For this review, take the finished solid that the model builds, in its own axes (mm). A direction names the side the tool comes from. Coordinates: 2 decimals unless noted, no trailing zeros. Order: outer loops, then holes, each group sorted by start corner. A loop starts at its lowest first (then second) coordinate and runs counter-clockwise, first axis right, second up.
from build123d import *

# Parameters (mm, degrees)
BOSS_EXTRUDE1_DEPTH = 1.5
SKETCH2_W           = 0.621894726
SKETCH2_H           = 0.5
SKETCH3_W           = 0.313581939
SKETCH3_H           = 0.5
SKETCH4_W           = 0.917270519
SKETCH4_H           = 0.5
SKETCH5_W           = 0.282237083
SKETCH5_H           = 0.5
SKETCH6_W           = 0.605170604
SKETCH6_H           = 0.5


with BuildPart() as part:
    # Sketch1 → Boss-Extrude1 (new body)
    with BuildSketch(Plane(origin=(0, 0, 0), x_dir=(-1, 0, 0), z_dir=(0, 0, -1))):
        with BuildLine():
            Line((3.5, 1.5), (-3.5, 1.5))
            ThreePointArc((-3.5, 1.5), (-5, 0), (-3.5, -1.5))
            Line((-3.5, -1.5), (3.5, -1.5))
            ThreePointArc((3.5, -1.5), (5, 0), (3.5, 1.5))
        make_face()
    extrude(amount=-BOSS_EXTRUDE1_DEPTH)

    # Sketch2 → Revolve1 (revolve)
    with BuildSketch(Plane.XZ, mode=Mode.PRIVATE) as revolve1_sk:
        with Locations((3.731030185, 1.75)):
            Rectangle(SKETCH2_W, SKETCH2_H)
    revolve(revolve1_sk.sketch.rotate(Axis((3.420082822, 0, 2), (0, 0, -1)), 180), axis=Axis((3.420082822, 0, 2), (0, 0, -1)))

    # Sketch3 → Revolve2 (revolve)
    with BuildSketch(Plane.XZ, mode=Mode.PRIVATE) as revolve2_sk:
        with Locations((2.315287044, 1.75)):
            Rectangle(SKETCH3_W, SKETCH3_H)
    revolve(revolve2_sk.sketch.rotate(Axis((2.158496075, 0, 2), (0, 0, -1)), 180), axis=Axis((2.158496075, 0, 2), (0, 0, -1)))

    # Sketch4 → Revolve3 (revolve)
    with BuildSketch(Plane.XZ, mode=Mode.PRIVATE) as revolve3_sk:
        with Locations((0.45863526, 1.75)):
            Rectangle(SKETCH4_W, SKETCH4_H)
    revolve(revolve3_sk.sketch.rotate(Axis((0, 0, 2), (0, 0, -1)), 180), axis=Axis((0, 0, 2), (0, 0, -1)))

    # Sketch5 → Revolve4 (revolve)
    with BuildSketch(Plane.XZ.offset(0.093633391), mode=Mode.PRIVATE) as revolve4_sk:
        with Locations((-1.554138651, 1.75)):
            Rectangle(SKETCH5_W, SKETCH5_H)
    revolve(revolve4_sk.sketch.rotate(Axis((-1.695257192, -0.093633391, 2), (0, 0, -1)), 180), axis=Axis((-1.695257192, -0.093633391, 2), (0, 0, -1)))

    # Sketch6 → Revolve5 (revolve)
    with BuildSketch(Plane.XZ.offset(0.093633391), mode=Mode.PRIVATE) as revolve5_sk:
        with Locations((-2.693683223, 1.75)):
            Rectangle(SKETCH6_W, SKETCH6_H)
    revolve(revolve5_sk.sketch.rotate(Axis((-2.996268525, -0.093633391, 2), (0, 0, -1)), 180), axis=Axis((-2.996268525, -0.093633391, 2), (0, 0, -1)))


solid = part.part
1. Take a section at A-A, the plane x = 0. Give the boundary of the cut face in (y, z).
Answer below:
outline: (-1.5, 0) - (1.5, 0) - (1.5, 1.5) - (0.92, 1.5) - (0.92, 2) - (-0.92, 2) - (-0.92, 1.5) - (-1.5, 1.5) - close
2. Take a section at D-D, the plane x = 1.25. Give the boundary of the cut face in (y, z).
Answer below:
outline: (-1.5, 0) - (1.5, 0) - (1.5, 1.5) - (-1.5, 1.5) - close
3. Take a section at C-C, the plane z = 0.4. Give the boundary of the cut face in (x, y), plus the area to 3 significant figures.
Answer below:
outline: (-3.5, -1.5) - (3.5, -1.5) arc R1.5 ccw to (3.5, 1.5) - (-3.5, 1.5) arc R1.5 ccw to start
area: 28.1 mm2
4. The part is to be moulded in two halves that separate along X. For faces 3 (the face through (-3, 0, 2)), 4 (the face through (-3.573, 0.088, 1.754)), 5 (the face through (5, 0, 1)), say which applies: +X half, -X half, draft (parallel to the pull), parting line (faces both ways), or undercut.
Answer below:
face 3: draft
face 4: undercut
face 5: +X half
5. Machinability: for faces 1 (the face through (-0.875, 0.276, 1.754)), 2 (the face through (0, -1.5, 1)), which of the approach directions +Z, -Z, +X, -X, +Y, -Y give a long, thin tool a straight path to every point of the face, cutting with its end or side? Answer none if there is none.
Answer below:
face 1: +Z
face 2: +Z, -Z, +X, -X, -Y
6. Take a section at B-B, the plane y = 0. Give the boundary of the cut face in (x, z), plus the area to 3 significant figures.
Answer below:
outline: (-5, 0) - (5, 0) - (5, 1.5) - (4.04, 1.5) - (4.04, 2) - (2.8, 2) - (2.8, 1.5) - (2.47, 1.5) - (2.47, 2) - (1.84, 2) - (1.84, 1.5) - (0.92, 1.5) - (0.92, 2) - (-0.92, 2) - (-0.92, 1.5) - (-1.43, 1.5) - (-1.43, 2) - (-1.96, 2) - (-1.96, 1.5) - (-2.4, 1.5) - (-2.4, 2) - (-3.59, 2) - (-3.59, 1.5) - (-5, 1.5) - close
area: 17.7 mm2
7. To check wall thickness, follow L1, parallel to Z at x = -1, y = -0.9; L2, parallel to Y at x = 0.75, z = 1.7; L3, parallel to X at y = -0.3, z = 1.15. State the ranges of each line that lie inside material, in increasing order.
Answer below:
L1: z = 0 to 1.5
L2: y = -0.53 to 0.53
L3: x = -4.97 to 4.97
